Answer from the drawing. Dimensions are ordinates in mm from the lowest x, y and z of the part. A direction names the side the tool comes from. Coordinates: 2 decimals unless noted, no trailing zeros. Order: outer loops, then holes, each group sorted by start corner. A loop starts at its lowest first (then second) coordinate and runs counter-clockwise, first axis right, second up. Notation, with made-up numbers: (35, 60) -> (57, 60) arc R16 ccw to (57, 90) -> close; hole circle Ø11 at (22.5, 83.25). An arc over 180 degrees is marked (long way). Answer in a Markdown table with one row per item.
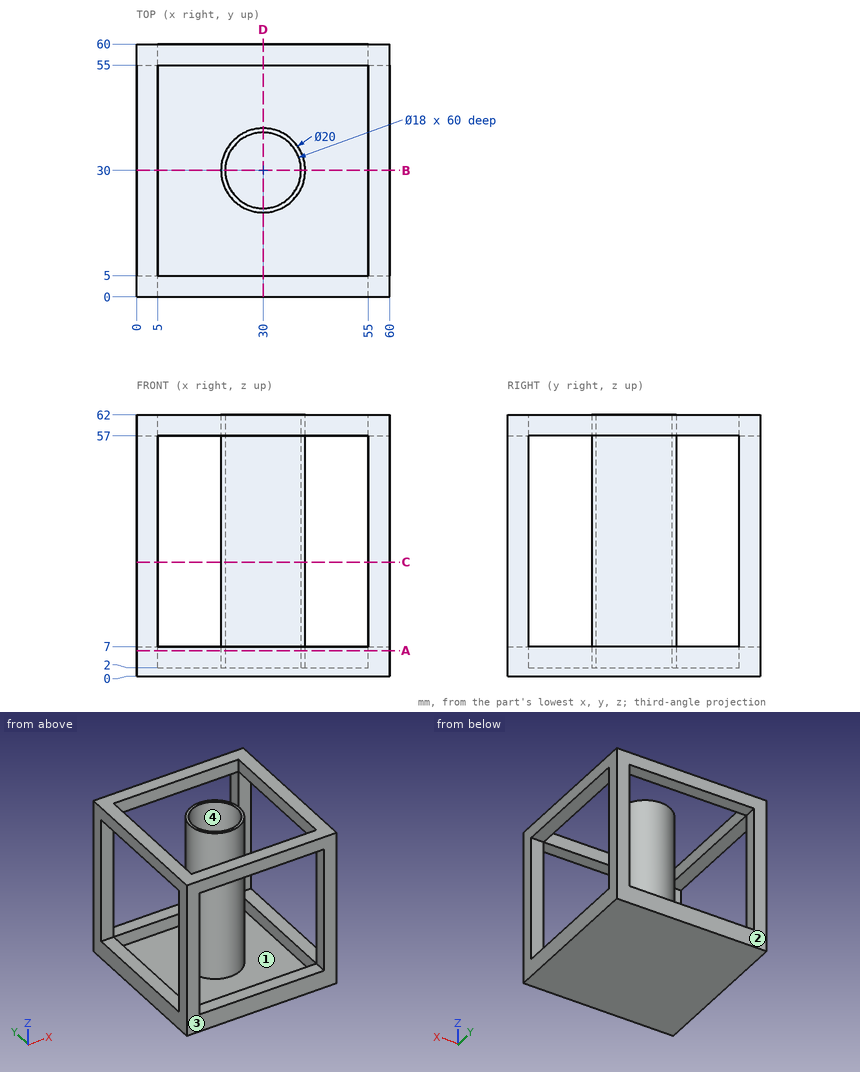
(1) Which of the six approach directions +Z, -Z, +X, -X, +Y, -Y give full straight-line access (tool end or side, diameter ignored) to the marked faces 1 and 2?
Check values:
| item | result |
|---|---|
| face 1 | +Z |
| face 2 | +Z, -Z, +X, -X, +Y |
(2) Flat-ended cylindrical pins translate along their axes: pin 1 (4 mm diameter, centred on y = 20, z = 31.5, fed in from +X); pin 2 (5 mm diameter, centred on x = 21.5, z = 26, fed in from -Y); pin 3 (1 mm diameter, centred on x = 14, y = 36, fed in from +Z). Find the tip coordinate at first contact, or state that the pin passes through.
Check values:
| item | result |
|---|---|
| pin 1 | x = 36 |
| pin 2 | y = 22 |
| pin 3 | z = 2 |
(3) A cutting plane is placed at C-C, the plane z = 27. Determine the outline of the cut face in (x, y).
Check values:
| item | result |
|---|---|
| outline | (0, 0) -> (5, 0) -> (5, 5) -> (0, 5) -> close; (0, 55) -> (5, 55) -> (5, 60) -> (0, 60) -> close; circle Ø20 at (30, 30); (55, 0) -> (60, 0) -> (60, 5) -> (55, 5) -> close; (55, 55) -> (60, 55) -> (60, 60) -> (55, 60) -> close; hole circle Ø18 at (30, 30) |
(4) A cutting plane is placed at A-A, the plane z = 6. Determine the outline of the cut face in (x, y), then the cut area to 3 significant figures.
Check values:
| item | result |
|---|---|
| outline | (0, 0) -> (60, 0) -> (60, 60) -> (0, 60) -> close; circle Ø20 at (30, 30); hole (5, 5) -> (55, 5) -> (55, 55) -> (5, 55) -> close; hole circle Ø18 at (30, 30) |
| area | 1,160 mm² |
(5) For a pull along X with two mould halves and no side action, classify the marked faces 3 and 4 as released by +X, released by -X, zero draft, split by the parting line, or undercut.
Check values:
| item | result |
|---|---|
| face 3 | zero draft |
| face 4 | undercut |
(6) A cutting plane is placed at B-B, the plane y = 30. Determine the outline of the cut face in (x, z).
Check values:
| item | result |
|---|---|
| outline | (0, 0) -> (60, 0) -> (60, 7) -> (55, 7) -> (55, 2) -> (40, 2) -> (40, 62) -> (39, 62) -> (39, 2) -> (21, 2) -> (21, 62) -> (20, 62) -> (20, 2) -> (5, 2) -> (5, 7) -> (0, 7) -> close; (0, 57) -> (5, 57) -> (5, 62) -> (0, 62) -> close; (55, 57) -> (60, 57) -> (60, 62) -> (55, 62) -> close |
(7) Find the intervals of material crossed by line 1 along Z through (x, y) = (28.5, 4.5); line 2 along Y through (x, z) = (30, 23); line 3 along X through (y, z) = (57, 53.5), in increasing order. Write a range as from..to.
Check values:
| item | result |
|---|---|
| line 1 | 0..7, 57..62 |
| line 2 | 20..21, 39..40 |
| line 3 | 0..5, 55..60 |
